Input: part model. Units: mm. Frame: model coordinates. Round coordinates to 2 decimals unless told otherwise and drop trailing zeros. Loops run counter-clockwise (first coordinate to the right, second up) from the corner with the lowest first, then second, coordinate; pieces in that order, holes last. Notation, with made-up numbers: M -26.5,71 L 31.5,71 A23 ccw 31.5,88 Z; hole C 47,42 d5. An arc over 180 degrees is marked long. Return JSON: item names as keys, results as strings. Group by question number.
1) Contact query for flat-ended pins moving along their axis: P1, Ø2, axis at x = 0.5, y = 4, coming from the +Z side; P2, Ø1.7, axis at x = -4, z = 0, coming from the +Y side; P3, Ø5, axis at x = 2, z = -4.5, coming from the +Y side. Output: stop coordinate, or through.
2) Section B-B (y = 4.15). Output: boundary loops of the cut face in (x, z), plus the area to 3 significant figures.
3) Section A-A (y = 2.65). Output: boundary loops of the cut face in (x, z).
4) Mould query, pull axis X, two halves, no side actions, for faces 1 (the face through (0, 0, 3)), 2 (the face through (0.911, 2.282, 1.693)), 3 (the face through (2.3, 4.28, -0.72)). Classes: +X half, -X half, draft (parallel to the pull), parting line (faces both ways), or undercut.
5) Material intervals for line 1 (Z direction, x = -1.25, y = 2.05); line 2 (Z direction, x = 1.5, y = 1.8); line 3 (Y direction, x = -2, z = -1), sorted ascending. Write a range as from..to.
from build123d import *

# Parameters (mm, degrees)
SKETCH1_R           = 6
BOSS_EXTRUDE1_DEPTH = 4.5
BOSS_EXTRUDE1_TAPER = 40
CUT_EXTRUDE1_DEPTH  = 5
SKETCH5_R           = 0.75
CUT_EXTRUDE2_DEPTH  = 5


with BuildPart() as part:
    # Sketch1 → Boss-Extrude1 (new body)
    with BuildSketch(Plane(origin=(0, 0, 0), x_dir=(1, 0, 0), z_dir=(0, 1, 0))):
        Circle(SKETCH1_R)
    extrude(amount=BOSS_EXTRUDE1_DEPTH, taper=BOSS_EXTRUDE1_TAPER)

    # Sketch3 → Cut-Extrude1 (cut)
    with BuildSketch(Plane(origin=(0, 4.5, 0), x_dir=(1, 0, 0), z_dir=(0, 1, 0))):
        Polygon((0, 2.25), (-0.509878041, 1.569243252), (-1.322516818, 1.820288237), (-1.334878041, 0.969845666), (-2.139877162, 0.695288237), (-1.65, 0), (-2.139877162, -0.695288237), (-1.334878041, -0.969845666), (-1.322516818, -1.820288237), (-0.509878041, -1.569243252), (0, -2.25), (0.509878041, -1.569243252), (1.322516818, -1.820288237), (1.334878041, -0.969845666), (2.139877162, -0.695288237), (1.65, 0), (2.139877162, 0.695288237), (1.334878041, 0.969845666), (1.322516818, 1.820288237), (0.509878041, 1.569243252), align=None)
    extrude(amount=-CUT_EXTRUDE1_DEPTH, mode=Mode.SUBTRACT)

    # Sketch5 → Cut-Extrude2 (cut)
    with BuildSketch(Plane.XZ):
        with Locations(Location((4, 0, 0), (0, 0, 270))):
            Circle(SKETCH5_R)
        with Locations(Location((-4, 0, 0), (0, 0, 270))):
            Circle(SKETCH5_R)
    extrude(amount=-CUT_EXTRUDE2_DEPTH, mode=Mode.SUBTRACT)


solid = part.part
Returned:
{
 "1": {"P1": "stops at z = 3.46", "P2": "stops at y = 3.4", "P3": "stops at y = 4.26"},
 "2": {"outline": "C 0,0 d5.04; hole M -2.14,-0.7 L -1.33,-0.97 L -1.32,-1.82 L -0.51,-1.57 L 0,-2.25 L 0.51,-1.57 L 1.32,-1.82 L 1.33,-0.97 L 2.14,-0.7 L 1.65,0 L 2.14,0.7 L 1.33,0.97 L 1.32,1.82 L 0.51,1.57 L 0,2.25 L -0.51,1.57 L -1.32,1.82 L -1.33,0.97 L -2.14,0.7 L -1.65,0 Z", "area": "8.44 mm^2"},
 "3": {"outline": "M -3.71,-0.69 A3.78 ccw 3.71,-0.69 A0.75 cw 3.71,0.69 A3.78 ccw -3.71,0.69 A0.75 cw Z; hole M -2.14,-0.7 L -1.33,-0.97 L -1.32,-1.82 L -0.51,-1.57 L 0,-2.25 L 0.51,-1.57 L 1.32,-1.82 L 1.33,-0.97 L 2.14,-0.7 L 1.65,0 L 2.14,0.7 L 1.33,0.97 L 1.32,1.82 L 0.51,1.57 L 0,2.25 L -0.51,1.57 L -1.32,1.82 L -1.33,0.97 L -2.14,0.7 L -1.65,0 Z"},
 "4": {"face 1": "draft", "face 2": "undercut", "face 3": "parting line"},
 "5": {"line 1": "z = -4.09..-1.8, 1.8..4.09", "line 2": "z = -4.23..-0.91, 0.91..4.23", "line 3": "y = 0..4.49"}
}
